Verification items for this drawing (mm, ordinates from the low corner). A direction names the side the tool comes from. Coordinates: 2 decimals unless noted, no trailing zeros. Write each loop counter-clockwise with the first axis right and the second up, starting at its lowest first coordinate (ties: lowest second). Pieces come first, ordered by that corner, then holes.
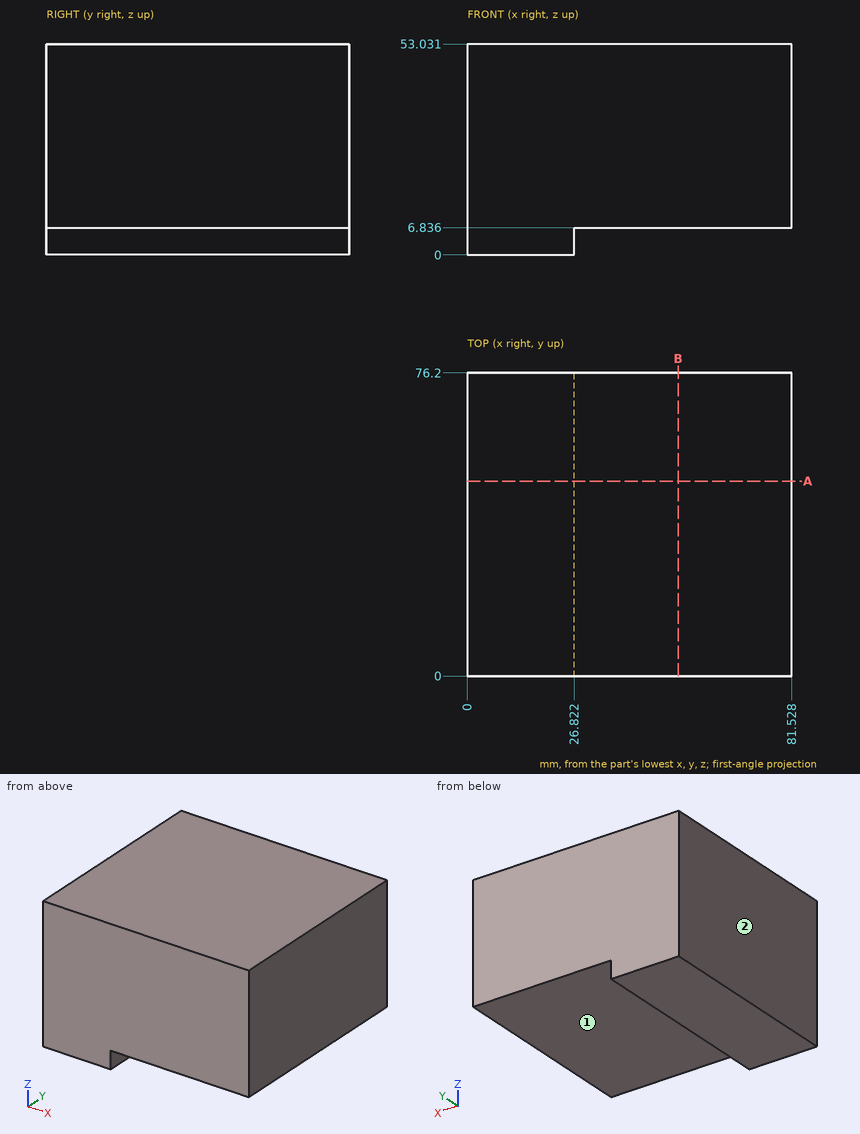
1. Sectioned sample at A-A, the plane y = 49. Record the boundary of the cut face in (x, z), and give its area (3 significant figures).
Computed values:
outline: (0, 0) - (26.82, 0) - (26.82, 6.84) - (81.53, 6.84) - (81.53, 53.03) - (0, 53.03) - close
area: 3,950 mm2
2. Thickness scan on line 1 along Z through (x, y) = (38, 67.5); line 2 along X through (y, z) = (30, 6.5). Record the ranges inside material, lowest first.
Computed values:
line 1: z = 6.84 to 53.03
line 2: x = 0 to 26.82
3. Gauge pin test, flat ends, axial feed: pin 1 Ø6 at (y, z) = (16, 22.5) entering from -X; pin 2 Ø7.5 at (y, z) = (51, 3) entering from +X. Record the tip position at first contact, or that the pin passes through.
Computed values:
pin 1: stops at x = 0
pin 2: stops at x = 26.82
4. Sectioned sample at B-B, the plane x = 53. Record the boundary of the cut face in (y, z).
Computed values:
outline: (0, 6.84) - (76.2, 6.84) - (76.2, 53.03) - (0, 53.03) - close
5. Access from +Z, -Z, +X, -X, +Y, -Y to the whole of each face (thin tool, end or side, straight path). Record for the marked faces 1 and 2.
Computed values:
face 1: -Z, +X, +Y, -Y
face 2: +Z, -Z, -X, +Y, -Y
